from build123d import *

# Parameters (mm, degrees)
BASE_DEPTH               = 46
BASE_DEPTH_BACK          = 46
SKETCH4_W                = 60
SKETCH4_H                = 69
LIDAR_DEPTH              = 41
LIDAR_DEPTH_BACK         = 46
HOLEFRONTBACK_DEPTH      = 66.941261741
HOLEFRONTBACK_DEPTH_BACK = 66.941261741
SKETCH6_W                = 82
SKETCH6_H                = 43
RAIL_START               = -30
RAIL_DEPTH               = 60
SKETCH8_R                = 1
RAILHOLE_DEPTH           = 71.740017959
LPATTERN1_COUNT          = 15
LPATTERN1_PITCH          = 3.71
FILLET2_R                = 4
SAFETY_REACH             = 72.74
SKETCH9_R                = 1
SAFETY_DIRECTION_2_DEPTH = 34.6
LPATTERN2_COUNT          = 9
LPATTERN2_PITCH          = 3.71


with BuildPart() as part:
    # Sketch4 → Base (new, two sides: drawn at the far end of the back side and taken through both)
    with BuildSketch(Plane(origin=(0, 0, 0), x_dir=(0, 0, -1), z_dir=(1, 0, 0)).offset(-BASE_DEPTH_BACK)):
        with Locations((0, -2)):
            Rectangle(SKETCH4_W, SKETCH4_H)
    extrude(amount=BASE_DEPTH + BASE_DEPTH_BACK)

    # Sketch5 → LIDAR (cut, two sides: drawn at the far end of the back side and taken through both)
    with BuildSketch(Plane(origin=(0, 0, 0), x_dir=(0, 0, -1), z_dir=(1, 0, 0)).offset(-LIDAR_DEPTH_BACK)):
        Polygon((-25, 27.5), (-25, 14.5), (-10.630657971, -32.5), (25, -32.5), (25, 27.5), align=None)
    extrude(amount=LIDAR_DEPTH + LIDAR_DEPTH_BACK, mode=Mode.SUBTRACT)

    # Sketch6 → HoleFrontBack (cut, two sides: drawn at the far end of the back side and taken through both)
    with BuildSketch(Plane.XY.offset(-HOLEFRONTBACK_DEPTH_BACK)):
        with Locations((0, -7)):
            Rectangle(SKETCH6_W, SKETCH6_H)
    extrude(amount=HOLEFRONTBACK_DEPTH + HOLEFRONTBACK_DEPTH_BACK, mode=Mode.SUBTRACT)

    # Sketch7 → Rail (add)
    with BuildSketch(Plane.XY.offset(RAIL_START)):
        Polygon((-9, -36.5), (9, -36.5), (11.335, -40.544338636), (9, -44.588677271), (-9, -44.588677271), (-11.335, -40.544338636), align=None)
    extrude(amount=RAIL_DEPTH)

    # Sketch8 → RailHole (cut, symmetric)
    with BuildSketch(Plane(origin=(0, 0, 0), x_dir=(0, 0, -1), z_dir=(1, 0, 0))):
        with Locations(Location((-26.29, -38.6, 0), (0, 0, 270))):
            Circle(SKETCH8_R)
    railhole = extrude(amount=RAILHOLE_DEPTH, both=True, mode=Mode.SUBTRACT)

    # LPattern1: RailHole ×15
    with Locations(*[(0, 0, -i * LPATTERN1_PITCH) for i in range(1, LPATTERN1_COUNT)]):
        add(railhole, mode=Mode.SUBTRACT)

    # Fillet2
    fillet2_edges = [part.edges().sort_by_distance(p)[0] for p in [
        (27.5, -36.5, -30),
        (27.5, -36.5, 30),
        (0, 32.5, 30),
        (0, 32.5, -30),
        (-27.5, -36.5, -30),
        (-27.5, -36.5, 30),
    ]]
    fillet(fillet2_edges, radius=FILLET2_R)

    # Safety: up to this face of the body (flat: up to its plane)
    safety_end = Plane(part.part.faces().sort_by_distance((0, 32.5, 0))[0])
    # Sketch9 → Safety (cut, up to the picked face)
    with BuildSketch(Plane(origin=(0, 0, 0), x_dir=(1, 0, 0), z_dir=(0, 1, 0)), mode=Mode.PRIVATE) as safety_sk1:
        with Locations(Location((-42.9, 22.29, 0), (0, 0, 270))):
            Circle(SKETCH9_R)
    safety_tool1 = split(extrude(safety_sk1.sketch, amount=SAFETY_REACH, mode=Mode.PRIVATE), bisect_by=safety_end, keep=Keep.BOTH, mode=Mode.PRIVATE)
    safety = safety_tool1.solids().sort_by(Axis((-42.9, 0, -22.29), (0, 1, 0)))[0]
    add(safety, mode=Mode.SUBTRACT)

    # Sketch9 → Safety direction 2 (cut)
    with BuildSketch(Plane(origin=(0, 0, 0), x_dir=(1, 0, 0), z_dir=(0, 1, 0))):
        with Locations(Location((-42.9, 22.29, 0), (0, 0, 270))):
            Circle(SKETCH9_R)
    safety_direction_2 = extrude(amount=-SAFETY_DIRECTION_2_DEPTH, mode=Mode.SUBTRACT)

    # LPattern2: Safety, Safety direction 2 ×9
    with Locations(*[(0, 0, i * LPATTERN2_PITCH) for i in range(1, LPATTERN2_COUNT)]):
        add(safety, mode=Mode.SUBTRACT)
        add(safety_direction_2, mode=Mode.SUBTRACT)


solid = part.part
Design review of the part built by this model. Coordinates are the model's own, in mm. A direction names the side the tool comes from. Round coordinates to 2 decimals unless told otherwise and drop trailing zeros. Loops run counter-clockwise (first coordinate to the right, second up) from the corner with the lowest first, then second, coordinate; pieces in that order, holes last. Notation, with made-up numbers: (-0.5, 74) - (46.5, 74) arc R17 cw to (46.5, 91) - close; hole circle Ø6 at (2.5, -38). An arc over 180 degrees is marked (long way). One line per item, written item: value. Start each with the question number.
1) For faces 1 (the cylindrical face through (0.644, 31.359, -28.797)), 2 (the flat face through (-13, 17, -25)), 3 (the flat face through (-41, -7, -28)), 4 (the flat face through (41, -3, 0)), 5 (the flat face through (0, -44.589, 0)), list the 3-axis set-ups (+Z, -Z, +X, -X, +Y, -Y) from which the entire face can be reached by the end or side of a thin tool; tool diameter is ignored.
2) Consider section B-B on y = -18. Give the boundary of the cut face in (x, z), then the cut area to 3 significant figures.
3) Insertion check: pin 1 Ø1.6 at (x, z) = (-42.9, 7.39) entering from +Y; pin 2 Ø1.5 at (y, z) = (-12.5, -7) entering from -X; pin 3 Ø1.2 at (x, z) = (-42.9, -18.58) entering from -Y; pin 4 Ø1.8 at (y, z) = (-38.6, 22.58) entering from -X. Each pin has a flat end and moves straight along its axis. Give the tip position at first contact, or say it passes through.
4) Draft analysis for pull direction X (two halves, no side actions). For faces 6 (the flat face through (-46, -1.5, 20.4)), 7 (the flat face through (27, -36.5, 0)), 8 (the flat face through (-1, 14.5, -28)), state which applies: +X half, -X half, draft (parallel to the pull), parting line (faces both ways), or undercut.
5) Consider section C-C on y = -1. Give the boundary of the cut face in (x, z).
6) Consider section A-A on x = -19. Give the boundary of the cut face in (y, z), then the cut area to 3 significant figures.
7) To check wall thickness, follow L1, parallel to Y at x = 2, z = 15; L2, parallel to X at y = 29.65, z = -14.87; L3, parallel to Y at x = 10, z = 26. State the ranges of each line that lie inside material, in increasing order. Write a range as from..to.
Reported:
1. face 1: -Z, +X, -X, +Y
1. face 2: -X
1. face 3: +Z, -Z
1. face 4: none
1. face 5: +Z, -Z, +X, -X, -Y
2. outline: (-46, -30) - (-41, -30) - (-41, -25) - (-46, -25) - close; (-46, 15.06) - (-41, 15.06) - (-41, 30) - (-46, 30) - close; (41, -30) - (46, -30) - (46, 30) - (41, 30) - close
2. area: 400 mm^2
3. pin 1: stops at y = -34.6
3. pin 2: stops at x = 41
3. pin 3: stops at y = -36.5
3. pin 4: passes through
4. face 6: -X half
4. face 7: draft
4. face 8: undercut
5. outline: (-46, -30) - (-41, -30) - (-41, -25) - (-46, -25) - close; (-46, 20.26) - (-41, 20.26) - (-41, 30) - (-46, 30) - close; (41, -30) - (46, -30) - (46, 30) - (41, 30) - close
6. outline: (-36.5, -26) arc R4 ccw to (-32.5, -30) - (-28.5, -30) - (-28.5, -25) - (-32.5, -25) - (-32.5, 10.63) - (-28.5, 11.85) - (-28.5, 30) - (-32.5, 30) arc R4 ccw to (-36.5, 26) - close; (14.5, -30) - (28.5, -30) arc R4 ccw to (32.5, -26) - (32.5, 26) arc R4 ccw to (28.5, 30) - (14.5, 30) - (14.5, 25) - (27.5, 25) - (27.5, -25) - (14.5, -25) - close
6. area: 751 mm^2
7. L1: y = -44.59..-39.59, -37.61..-28.5, 27.5..32.5
7. L2: x = -46..-43.9, -41.9..46
7. L3: y = -42.86..-39.56, -36.5..-28.5, 14.5..32.5
